```python
from build123d import *

# Parameters (mm, degrees)
SKETCH1_R           = 3.125
BOSS_EXTRUDE1_DEPTH = 5.8
FILLET1_R           = 1


with BuildPart() as part:
    # Sketch1 → Boss-Extrude1 (new body)
    with BuildSketch(Plane(origin=(0, 0, 0), x_dir=(1, 0, 0), z_dir=(0, 1, 0))):
        with BuildLine():
            Line((-1.75, 10), (-3.75, 10))
            Line((-3.75, 10), (-3.75, -18))
            ThreePointArc((-3.75, -18), (9.742495495, -21.686970301), (0, -11.65078745))
            ThreePointArc((0, -11.65078745), (-0.926705166, -12.258329392), (-1.75, -13))
            Line((-1.75, -13), (-1.75, -3.31662479))
            ThreePointArc((-1.75, -3.31662479), (-0.901431372, -3.640044159), (0, -3.75))
            ThreePointArc((0, -3.75), (3.640044159, 0.901431372), (-1.75, 3.31662479))
            Line((-1.75, 3.31662479), (-1.75, 10))
        make_face()
        with Locations(Location((0, 0, 0), (0, 0, 270))):
            Circle(SKETCH1_R, mode=Mode.SUBTRACT)
    extrude(amount=BOSS_EXTRUDE1_DEPTH)

    # Fillet1
    fillet1_edges = [part.edges().sort_by_distance(p)[0] for p in [
        (-3.75, 2.9, -10),
    ]]
    fillet(fillet1_edges, radius=FILLET1_R)


solid = part.part
```
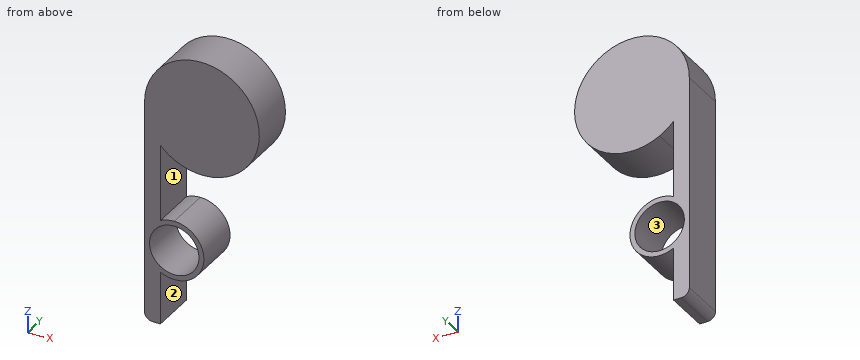
Source: CAD feature listing. Evaluate the final solid. Frame: model axes, mm. Face numbers are marked on the shaded views. Give positions to 0.01 mm unless a question says otherwise; leave off trailing zeros. Order: outer loops, then holes, each group sorted by start corner. A loop starts at its lowest first (then second) coordinate and runs counter-clockwise, first axis right, second up.
(1) Section query C-C (x = 2.5). Return the cut outline in (y, z) (3 decimals).
(2) Section query B-B (z = 12). Return the cut outline in (x, y).
(3) Section query D-D (z = 6). Return the cut outline in (x, y).
(4) Contact query for flat-ended pins moving along their axis: P1, Ø2, axis at x = 7, y = 3, coming from the -Z side; P2, Ø1.7, axis at y = 3, z = -5.5, coming from the +X side; P3, Ø2, axis at x = 4, y = 4.5, coming from the +Z side. Output: stop coordinate, or through.
(5) Section query A-A (y = 4.9). Return the cut outline in (x, z) (3 decimals), plus the area to 3 significant figures.
(6) Material intervals for line 1 along X through (y, z) = (4.5, 0) (3 decimals); line 2 along Z through (x, y) = (3.25, 5.45); line 3 along X through (y, z) = (0.5, -5), sorted ascending.
(7) Pull-direction query (Z, two-part tool) for the marked faces 1, 2 and 3; classes: +Z half, -Z half, draft (parallel to the pull), parting line (faces both ways), or undercut.
Outcome:
1. outline: (0, -2.795) - (5.8, -2.795) - (5.8, -1.875) - (0, -1.875) - close; (0, 1.875) - (5.8, 1.875) - (5.8, 2.795) - (0, 2.795) - close; (0, 10.819) - (5.8, 10.819) - (5.8, 25.181) - (0, 25.181) - close
2. outline: (-3.75, 0) - (-1.75, 0) - (-1.75, 5.8) - (-3.75, 5.8) - close; (-0.57, 0) - (7.57, 0) - (7.57, 5.8) - (-0.57, 5.8) - close
3. outline: (-3.75, 0) - (-1.75, 0) - (-1.75, 5.8) - (-3.75, 5.8) - close
4. P1: stops at z = 11.19
4. P2: stops at x = -1.75
4. P3: stops at z = 25.25
5. outline: (-3.75, -9) arc R1 ccw to (-2.75, -10) - (-1.75, -10) - (-1.75, -3.317) arc R3.75 ccw (long way) to (-1.75, 3.317) - (-1.75, 13) arc R7.25 ccw (long way) to (-3.75, 18) - close; hole circle Ø6.25 at (0, 0)
5. area: 218 mm2
6. line 1: x = -3.75 to -3.125, 3.125 to 3.75
6. line 2: z = -1.87 to 1.87, 10.75 to 25.25
6. line 3: x = -3.75 to -1.75
7. face 1: undercut
7. face 2: draft
7. face 3: undercut
